The figure shows three views and two pictorial views of one solid part (mm, origin at its lowest corner). Answer the questions. A direction names the side the tool comes from. Round coordinates to 2 decimals unless told otherwise and drop trailing zeros. Order: outer loops, then holes, each group sorted by start corner. A loop starts at its lowest first (then second) coordinate and runs counter-clockwise, first axis right, second up. Notation, with made-up numbers: (-12, 69) - (36, 69) arc R37 ccw to (36, 105) - close; hole circle Ø5 at (38, 22.25). An arc over 180 degrees is marked (long way). Write item = value, one per line.
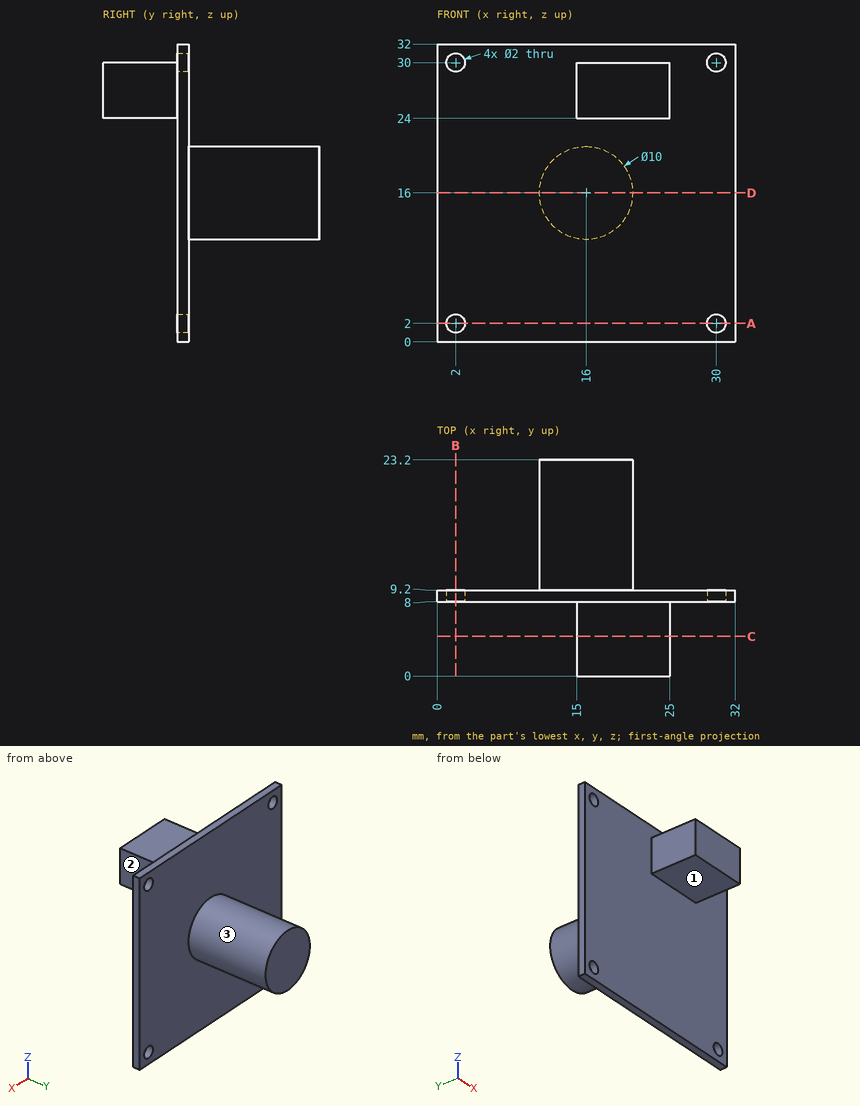
Q1. Flat-ended cylindrical pins translate along their axes: P1, Ø5, axis at x = 14, y = 18, coming from the +Z side; P2, Ø2.5, axis at x = 18.5, y = 4.5, coming from the -Z side; P3, Ø1.8, axis at y = 4, z = 27, coming from the +X side. Find the tip coordinate at first contact, or state that the pin passes through.
Model answer:
P1 = 21
P2 = 24
P3 = 25
Q2. For the marked faces 1, 2 and 3, determine the directions among +Z, -Z, +X, -X, +Y, -Y from which every point of the face is accessible in a straight line to the end or side of a thin tool.
Model answer:
face_1 = -Z, +X, -X, -Y
face_2 = +Z, -Z, +X, -Y
face_3 = +Y
Q3. Section C-C on y = 4.25 is taken. Determine the outline of the cut face in (x, z).
Model answer:
outline = (15, 24) - (25, 24) - (25, 30) - (15, 30) - close
Q4. Section B-B on x = 2 is taken. Determine the outline of the cut face in (y, z).
Model answer:
outline = (8, 0) - (9.2, 0) - (9.2, 1) - (8, 1) - close; (8, 3) - (9.2, 3) - (9.2, 29) - (8, 29) - close; (8, 31) - (9.2, 31) - (9.2, 32) - (8, 32) - close
Q5. Find the intervals of material crossed by line 1 (X direction, y = 8.95, z = 30); line 2 (Y direction, x = 2.5, z = 3.5); line 3 (Y direction, x = 21, z = 29.5), in increasing order. Write a range as from..to.
Model answer:
line_1 = 0..1, 3..29, 31..32
line_2 = 8..9.2
line_3 = 0..9.2
Q6. Section A-A on z = 2 is taken. Determine the outline of the cut face in (x, y).
Model answer:
outline = (0, 8) - (1, 8) - (1, 9.2) - (0, 9.2) - close; (3, 8) - (29, 8) - (29, 9.2) - (3, 9.2) - close; (31, 8) - (32, 8) - (32, 9.2) - (31, 9.2) - close
Q7. Section D-D on z = 16 is taken. Determine the outline of the cut face in (x, y), then the cut area to 3 significant figures.
Model answer:
outline = (0, 8) - (32, 8) - (32, 9.2) - (21, 9.2) - (21, 23.2) - (11, 23.2) - (11, 9.2) - (0, 9.2) - close
area = 178 mm^2
